Check sheet for the modelled part. Datum: model origin and axes. Units: mm. Face numbers are marked on the shaded views. Round coordinates to 2 decimals unless told otherwise and drop trailing zeros. Write each loop counter-clockwise with the first axis right and the second up, starting at its lowest first coordinate (ties: lowest second). Pieces come first, ordered by that corner, then holes. Notation, with made-up numbers: M -17.5,-28 L 20.5,-28 A21 cw 20.5,-10 Z; hole C 49,62 d1. An arc over 180 degrees is marked long. Answer in a Markdown table with one row per item.
```python
from build123d import *

# Parameters (mm, degrees)
SKETCH1_R           = 82.55
SKETCH1_R_2         = 76.2
BOSS_EXTRUDE1_DEPTH = 1219.2
SKETCH2_R           = 1.5875
CUT_EXTRUDE1_DEPTH  = 1225.77656942
CIRPATTERN1_COUNT   = 6


with BuildPart() as part:
    # Sketch1 → Boss-Extrude1 (new, symmetric)
    with BuildSketch(Plane(origin=(0, 0, 0), x_dir=(1, 0, 0), z_dir=(0, 1, 0))):
        with Locations(Location((0, 0, 0), (0, 0, 270))):
            Circle(SKETCH1_R)
        with Locations(Location((0, 0, 0), (0, 0, 270))):
            Circle(SKETCH1_R_2, mode=Mode.SUBTRACT)
    extrude(amount=BOSS_EXTRUDE1_DEPTH, both=True)

    # Sketch2 → Cut-Extrude1 (cut, through all)
    with BuildSketch(Plane(origin=(0, 0, 0), x_dir=(0, 0, -1), z_dir=(1, 0, 0))):
        with Locations((0, 1212.85)):
            Circle(SKETCH2_R)
    cut_extrude1 = extrude(amount=-CUT_EXTRUDE1_DEPTH, mode=Mode.SUBTRACT)

    # CirPattern1: Cut-Extrude1 ×6 about axis
    cirpattern1_axis = Axis((0, 1219.2, 0), (0, 1, 0))
    for i in range(1, CIRPATTERN1_COUNT):
        add(cut_extrude1.rotate(cirpattern1_axis, i * 360 / CIRPATTERN1_COUNT), mode=Mode.SUBTRACT)


solid = part.part
```
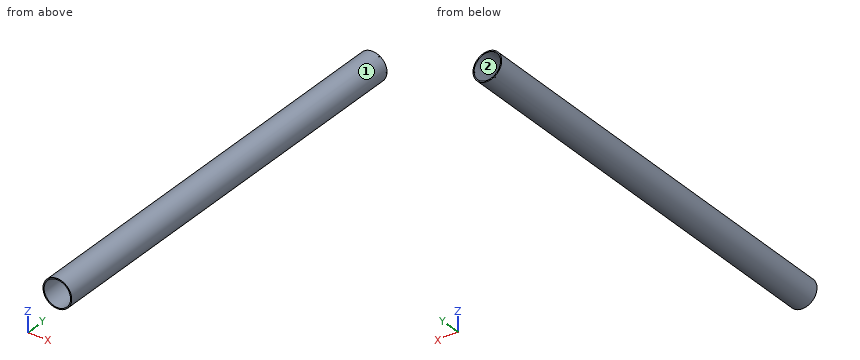
1. Section check C-C, the plane y = -734. Record the cut outline in (x, z).
Found:
| item | result |
|---|---|
| outline | C 0,0 d165.1; hole C 0,0 d152.4 |
2. Draft check along Z on the marked faces 1 and 2. Enter one of: +Z half, -Z half, draft (parallel to the pull), parting line (faces both ways), or undercut.
Found:
| item | result |
|---|---|
| face 1 | parting line |
| face 2 | undercut |
3. Section check B-B, the plane z = 36. Record the cut outline in (x, y), and give its area (3 significant figures).
Found:
| item | result |
|---|---|
| outline | M -74.29,-1219.2 L -67.16,-1219.2 L -67.16,1219.2 L -74.29,1219.2 Z; M 67.16,-1219.2 L 74.29,-1219.2 L 74.29,1219.2 L 67.16,1219.2 Z |
| area | 34,800 mm2 |
4. Go/stop test with flat-tipped pins: pin 1 (5 mm diameter, centred on x = 59, y = -403, fed in from +Z); pin 2 (1 mm diameter, centred on y = -630.5, z = -26.5, fed in from -X); pin 3 (5 mm diameter, centred on x = -28.5, y = 633, fed in from +Z); pin 4 (2.5 mm diameter, centred on y = 1212.85, z = 0, fed in from -X). Record where each tip stops, or that it passes through.
Found:
| item | result |
|---|---|
| pin 1 | stops at z = 60.19 |
| pin 2 | stops at x = -78.35 |
| pin 3 | stops at z = 78.35 |
| pin 4 | passes through |
5. Section check A-A, the plane x = 0. Record the cut outline in (y, z).
Found:
| item | result |
|---|---|
| outline | M -1219.2,-82.55 L 1219.2,-82.55 L 1219.2,-76.2 L -1219.2,-76.2 Z; M -1219.2,76.2 L 1219.2,76.2 L 1219.2,82.55 L -1219.2,82.55 Z |
6. Scan lines: L1, parallel to Y at x = 40, z = 69; L2, parallel to X at y = 691, z = -7; L3, parallel to Z at x = 4, y = -958.5. Record each from-to range of solid material in increasing order.
Found:
| item | result |
|---|---|
| L1 | y = -1219.2 to 1211.27, 1214.43 to 1219.2 |
| L2 | x = -82.25 to -75.88, 75.88 to 82.25 |
| L3 | z = -82.45 to -76.09, 76.09 to 82.45 |
